```python
from build123d import *

# Parameters (mm, degrees)
BOSS_EXTRUDE1_DEPTH            = 6.35
CUT_EXTRUDE1_DEPTH             = 7.35
F_2_5_2_5_DIAMETER_HOLE1_D     = 2.5
F_2_5_2_5_DIAMETER_HOLE1_DEPTH = 6.35
F_2_5_2_5_DIAMETER_HOLE2_D     = 2.5
F_2_5_2_5_DIAMETER_HOLE2_DEPTH = 6.35
F_4_2_4_2_DIAMETER_HOLE1_D     = 4.2
F_4_2_4_2_DIAMETER_HOLE1_DEPTH = 6.35
F_4_2_4_2_DIAMETER_HOLE2_D     = 4.2
F_4_2_4_2_DIAMETER_HOLE2_DEPTH = 6.35
F_4_2_4_2_DIAMETER_HOLE3_D     = 4.2
F_4_2_4_2_DIAMETER_HOLE3_DEPTH = 6.35
F_4_2_4_2_DIAMETER_HOLE4_D     = 4.2
F_4_2_4_2_DIAMETER_HOLE4_DEPTH = 6.35


with BuildPart() as part:
    # Sketch1 → Boss-Extrude1 (new body)
    with BuildSketch(Plane(origin=(0, 6.35, 0), x_dir=(1, 0, 0), z_dir=(0, 1, 0))):
        with BuildLine():
            Line((-15.289019905, 23.35), (-15.289019905, -7.15))
            ThreePointArc((-15.289019905, -7.15), (-14.11744703, -9.978427125), (-11.289019905, -11.15))
            Line((-11.289019905, -11.15), (11.288980095, -11.15))
            ThreePointArc((11.288980095, -11.15), (14.11740722, -9.978427125), (15.288980095, -7.15))
            Line((15.288980095, -7.15), (15.288980095, 23.35))
            Line((15.288980095, 23.35), (-15.289019905, 23.35))
        make_face()
        Polygon((-3.100095833, 15.4), (-3.100019905, 15.499999999), (-3.100019905, 21.85), (-3.09998206, 21.949999993), (3.099980095, 21.947653655), (3.099980095, 15.500000006), (3.100055965, 15.4), align=None, mode=Mode.SUBTRACT)
    extrude(amount=-BOSS_EXTRUDE1_DEPTH)

    # Sketch2 → Cut-Extrude1 (cut, through all)
    with BuildSketch(Plane.XZ):
        with BuildLine():
            Line((4.885014967, -7.854879297), (6.515054007, -9.484922393))
            ThreePointArc((6.515054007, -9.484922393), (9.484902488, -9.484926088), (9.484906183, -6.515077607))
            Line((9.484906183, -6.515077607), (7.854867143, -4.885034511))
            ThreePointArc((7.854867143, -4.885034511), (9.25, 0), (7.854867143, 4.885034511))
            Line((7.854867143, 4.885034511), (9.484906183, 6.515077607))
            ThreePointArc((9.484906183, 6.515077607), (9.484902486, 9.484926095), (6.515053997, 9.484922394))
            Line((6.515053997, 9.484922394), (4.885014967, 7.854879297))
            ThreePointArc((4.885014967, 7.854879297), (-1.1508e-05, 9.25), (-4.885034511, 7.854867143))
            Line((-4.885034511, 7.854867143), (-6.515097512, 9.484926088))
            ThreePointArc((-6.515097512, 9.484926088), (-9.484946, 9.484922391), (-9.484942299, 6.515073902))
            Line((-9.484942299, 6.515073902), (-7.854879297, 4.885014967))
            ThreePointArc((-7.854879297, 4.885014967), (-9.25, 0), (-7.854879297, -4.885014967))
            Line((-7.854879297, -4.885014967), (-9.484942298, -6.515073912))
            ThreePointArc((-9.484942298, -6.515073912), (-9.484945993, -9.484922393), (-6.515097512, -9.484926088))
            Line((-6.515097512, -9.484926088), (-4.885034511, -7.854867143))
            ThreePointArc((-4.885034511, -7.854867143), (-1.1508e-05, -9.25), (4.885014967, -7.854879297))
        make_face()
    extrude(amount=-CUT_EXTRUDE1_DEPTH, mode=Mode.SUBTRACT)

    # Ø2.5 (2.5) Diameter Hole1
    with Locations(Plane(origin=(0, 0, 0), x_dir=(-1, 0, 0), z_dir=(0, -1, 0))):
        with Locations((8.000019905, 18.675)):
            Hole(F_2_5_2_5_DIAMETER_HOLE1_D / 2, depth=F_2_5_2_5_DIAMETER_HOLE1_DEPTH)

    # Ø2.5 (2.5) Diameter Hole2
    with Locations(Plane(origin=(0, 0, 0), x_dir=(-1, 0, 0), z_dir=(0, -1, 0))):
        with Locations((-7.999980095, 18.675)):
            Hole(F_2_5_2_5_DIAMETER_HOLE2_D / 2, depth=F_2_5_2_5_DIAMETER_HOLE2_DEPTH)

    # Ø4.2 (4.2) Diameter Hole1
    with Locations(Plane(origin=(0, 0, 0), x_dir=(-1, 0, 0), z_dir=(0, -1, 0))):
        with Locations((-11.858647005, 11.5)):
            Hole(F_4_2_4_2_DIAMETER_HOLE1_D / 2, depth=F_4_2_4_2_DIAMETER_HOLE1_DEPTH)

    # Ø4.2 (4.2) Diameter Hole2
    with Locations(Plane(origin=(0, 0, 0), x_dir=(-1, 0, 0), z_dir=(0, -1, 0))):
        with Locations((11.858637076, 11.5)):
            Hole(F_4_2_4_2_DIAMETER_HOLE2_D / 2, depth=F_4_2_4_2_DIAMETER_HOLE2_DEPTH)

    # Ø4.2 (4.2) Diameter Hole3
    with Locations(Plane(origin=(0, 0, 0), x_dir=(-1, 0, 0), z_dir=(0, -1, 0))):
        with Locations((-11.859575542, -3.5)):
            Hole(F_4_2_4_2_DIAMETER_HOLE3_D / 2, depth=F_4_2_4_2_DIAMETER_HOLE3_DEPTH)

    # Ø4.2 (4.2) Diameter Hole4
    with Locations(Plane(origin=(0, 0, 0), x_dir=(-1, 0, 0), z_dir=(0, -1, 0))):
        with Locations((11.85956559, -3.500033723)):
            Hole(F_4_2_4_2_DIAMETER_HOLE4_D / 2, depth=F_4_2_4_2_DIAMETER_HOLE4_DEPTH)


solid = part.part
```
The listing builds one solid part. Answer for the finished solid, in the listing's coordinates (mm). A direction names the side the tool comes from. Coordinates: 2 decimals unless noted, no trailing zeros. Write each loop counter-clockwise with the first axis right and the second up, starting at its lowest first coordinate (ties: lowest second). Pieces come first, ordered by that corner, then holes. Notation, with made-up numbers: (89.5, 65.5) -> (132.5, 65.5) arc R21 ccw to (132.5, 85.5) -> close; hole circle Ø3 at (66.25, -37.5). An arc over 180 degrees is marked (long way). Write each question's results on one line, items separated by ' | '. Start each with the question number.
1) A cutting plane is placed at B-B (x = -2). Determine the outline of the cut face in (y, z), then the cut area to 3 significant figures.
2) A cutting plane is placed at D-D (y = 1.25). Count the separate pieces of the cut face and the enclosed holes in it, then the cut area to 3 significant figures.
3) A flat-ended cylindrical pin translates along its axis: pin 1 Ø2 at (x, z) = (1.5, -17.5) entering from -Y. Find the tip coordinate at first contact, or state that the pin passes through.
4) A tool of negligible diameter and unlimited length cuts with its end or side. For faces 1 (the cylindrical face through (14.086, 3.219, 10.009)), 2 (the cylindrical face through (-9.25, 3.13, 0.07)), from which of +Z, -Z, +X, -X, +Y, -Y can it reach the whole face along a straight path? Write none if from no direction.
5) A cutting plane is placed at C-C (x = -8.5). Determine the outline of the cut face in (y, z).
6) A cutting plane is placed at A-A (z = -11.5). Determine the outline of the cut face in (x, y).
7) For a pull along X with two mould halves and no side action, classify faces 3 (the cylindrical face through (-14.148, 3.219, 9.947)), 4 (the flat face through (15.289, 3, -8)), 5 (the flat face through (-8.68, 3.13, 5.71)) as +X half, -X half, draft (parallel to the pull), parting line (faces both ways), or undercut.
8) Straight lines are drawn through the part: probe 1 along X at (y, z) = (4.75, -11.5); probe 2 along Z at (x, y) = (-7, 3); probe 3 along Z at (x, y) = (-1, 1.75). For each, find the intervals that lie inside material, in ascending order.
Values follow:
1) outline: (0, -23.35) -> (6.35, -23.35) -> (6.35, -21.95) -> (0, -21.95) -> close; (0, -15.4) -> (6.35, -15.4) -> (6.35, -9.03) -> (0, -9.03) -> close; (0, 9.03) -> (6.35, 9.03) -> (6.35, 11.15) -> (0, 11.15) -> close | area: 62.8 mm²
2) separate pieces: 1 | enclosed holes: 8 | area: 610 mm²
3) pin 1: through
4) face 1: +Z, +X, +Y, -Y | face 2: +Y, -Y
5) outline: (0, -23.35) -> (6.35, -23.35) -> (6.35, -19.82) -> (0, -19.82) -> close; (0, -17.53) -> (6.35, -17.53) -> (6.35, -10.04) -> (0, -10.04) -> close; (0, -5.53) -> (6.35, -5.53) -> (6.35, -3.65) -> (0, -3.65) -> close; (0, 3.65) -> (6.35, 3.65) -> (6.35, 5.53) -> (0, 5.53) -> close; (0, 10.04) -> (6.35, 10.04) -> (6.35, 11.15) -> (0, 11.15) -> close
6) outline: (-15.29, 0) -> (-13.96, 0) -> (-13.96, 6.35) -> (-15.29, 6.35) -> close; (-9.76, 0) -> (9.76, 0) -> (9.76, 6.35) -> (-9.76, 6.35) -> close; (13.96, 0) -> (15.29, 0) -> (15.29, 6.35) -> (13.96, 6.35) -> close
7) face 3: -X half | face 4: +X half | face 5: undercut
8) probe 1: -15.29 to -13.96, -9.76 to 9.76, 13.96 to 15.29 | probe 2: -23.35 to -19.42, -17.93 to -9.85, 9.85 to 11.15 | probe 3: -23.35 to -21.95, -15.4 to -9.2, 9.2 to 11.15
